Read the model definition and answer for the solid it produces. Units are mm, in the model's axes. Face numbers are marked on the shaded views. A direction names the side the tool comes from. Coordinates: 2 decimals unless noted, no trailing zeros. Answer in a Markdown table with one row per item.
```python
from build123d import *

# Parameters (mm, degrees)
BOSS_EXTRUDE2_DEPTH       = 20
FILLET1_R                 = 30
FILLET2_R                 = 6
SKETCH2_R                 = 7
BOSS_EXTRUDE3_DEPTH       = 65.089952611
SKETCH3_R                 = 4.7625
CUT_EXTRUDE1_DEPTH        = 109.008396677
BOSS_EXTRUDE5_DEPTH       = 26.439795129
BOSS_EXTRUDE5_DEPTH_BACK  = 2
SKETCH6_R                 = 3
SKETCH8_R                 = 5
BOSS_EXTRUDE6_DEPTH       = 77
SKETCH9_R                 = 5
BOSS_EXTRUDE7_DEPTH       = 103.4
BOSS_EXTRUDE8_DEPTH       = 5
BOSS_EXTRUDE9_DEPTH       = 5
CUT_EXTRUDE2_DEPTH        = 2
BOSS_EXTRUDE14_START      = -1
BOSS_EXTRUDE14_DEPTH      = 3
BOSS_EXTRUDE15_DEPTH      = 15
SKETCH23_R                = 10
BOSS_EXTRUDE17_DEPTH      = 20
REVOLVE1_ANGLE            = 15
CIRPATTERN1_COUNT         = 4
CIRPATTERN1_ANGLE         = 273
SKETCH24_R                = 3.175
CUT_EXTRUDE3_DEPTH        = 25.4
SKETCH25_R                = 3.175
CUT_EXTRUDE4_DEPTH        = 25.4
BOSS_EXTRUDE20_DEPTH      = 1.5
BOSS_EXTRUDE20_DEPTH_BACK = 1.5
SKETCH26_W                = 46.97935404
SKETCH26_H                = 6


with BuildPart() as part:
    # Sketch1 → Boss-Extrude2 (new body)
    with BuildSketch(Plane.XY):
        Polygon((0, -8.361996352), (38.1, -8.361996352), (55.47415821, -26.885626298), (38.1, -33.761996352), (0, -33.761996352), (-17.37415821, -26.885626298), align=None)
    extrude(amount=BOSS_EXTRUDE2_DEPTH)

    # Fillet1
    fillet1_edges = [part.edges().sort_by_distance(p)[0] for p in [
        (0, -8.361996352, 10),
        (38.1, -8.361996352, 10),
    ]]
    fillet(fillet1_edges, radius=FILLET1_R)

    # Fillet2
    fillet2_edges = [part.edges().sort_by_distance(p)[0] for p in [
        (46.787079105, -30.323811325, 20),
        (-8.687079105, -30.323811325, 20),
        (46.787079105, -30.323811325, 0),
        (-8.687079105, -30.323811325, 0),
    ]]
    fillet(fillet2_edges, radius=FILLET2_R)

    # Sketch2 → Boss-Extrude3 (add)
    with BuildSketch(Plane.XZ.offset(33.761996352)):
        with Locations(Location((19.05, 10, 0), (0, 0, 180))):
            Circle(SKETCH2_R)
    extrude(amount=BOSS_EXTRUDE3_DEPTH)

    # Sketch3 → Cut-Extrude1 (cut, through all)
    with BuildSketch(Plane.XZ.offset(98.851948963)):
        with Locations((19.05, 10)):
            Circle(SKETCH3_R)
    extrude(amount=-CUT_EXTRUDE1_DEPTH, mode=Mode.SUBTRACT)

    # Sketch6 → Boss-Extrude5 (add, two sides: drawn at the far end of the back side and taken through both)
    with BuildSketch(Plane(origin=(16.71256452, -42.226747224, 0), x_dir=(-0.9298231117187001, -0.36800676748363437, 0), z_dir=(0.36800676748363437, -0.9298231117187001, 0)).offset(-BOSS_EXTRUDE5_DEPTH_BACK)):
        with Locations(Location((-32.344339698, -10, 0), (0, 0, 180))):
            Circle(SKETCH6_R)
    extrude(amount=BOSS_EXTRUDE5_DEPTH + BOSS_EXTRUDE5_DEPTH_BACK)

    # Sketch8 → Boss-Extrude6 (add)
    with BuildSketch(Plane(origin=(26.442588059, -66.811079804, 0), x_dir=(0.9298231117187001, 0.36800676748363437, 0), z_dir=(0.36800676748363437, -0.9298231117187001, 0))):
        with Locations((32.344339698, 10)):
            Circle(SKETCH8_R)
    extrude(amount=BOSS_EXTRUDE6_DEPTH)

    # Sketch9 → Boss-Extrude7 (add)
    with BuildSketch(Plane(origin=(-11.552720348, -29.189643592, 0), x_dir=(-0.9298231117187001, 0.36800676748363437, 0), z_dir=(-0.36800676748363437, -0.9298231117187001, 0))):
        with Locations(Location((-3.081920858, -10, 0), (0, 0, 53.130102354))):
            Circle(SKETCH9_R)
    extrude(amount=BOSS_EXTRUDE7_DEPTH)

    # Sketch11 → Boss-Extrude8 (add)
    with BuildSketch(Plane(origin=(32.698703106, -82.618072703, 0), x_dir=(-0.9298231117187001, -0.36800676748363437, 0), z_dir=(0.36800676748363437, -0.9298231117187001, 0))):
        with BuildLine():
            Line((-32.344339698, -3), (-22.259943936, -3))
            Line((-22.259943936, -3), (-22.259943936, -17))
            Line((-22.259943936, -17), (-32.344339698, -17))
            ThreePointArc((-32.344339698, -17), (-39.344339698, -10), (-32.344339698, -3))
        make_face()
    extrude(amount=BOSS_EXTRUDE8_DEPTH)

    # Sketch15 → Boss-Extrude9 (add)
    with BuildSketch(Plane(origin=(0, -68.851948963, 0), x_dir=(-1, 0, 0), z_dir=(0, -1, 0))):
        with BuildLine():
            Line((-19.05, -3), (-7.185808352, -3))
            Line((-7.185808352, -3), (-7.185808352, -17))
            Line((-7.185808352, -17), (-19.05, -17))
            ThreePointArc((-19.05, -17), (-26.05, -10), (-19.05, -3))
        make_face()
    extrude(amount=BOSS_EXTRUDE9_DEPTH)

    # Sketch17 → Cut-Extrude2 (cut)
    with BuildSketch(Plane(origin=(16.096305264, 15.097459572, 0), x_dir=(0, 0, -1), z_dir=(0.7293749969664987, 0.6841141087568068, 0))):
        with BuildLine():
            Line((-17, -51.560357903), (-17, -29.560357903))
            Line((-17, -29.560357903), (-3, -29.560357903))
            Line((-3, -29.560357903), (-3, -51.560357903))
            ThreePointArc((-3, -51.560357903), (-3.878679656, -53.681678246), (-6, -54.560357903))
            Line((-6, -54.560357903), (-14, -54.560357903))
            ThreePointArc((-14, -54.560357903), (-16.121320344, -53.681678246), (-17, -51.560357903))
        make_face()
    cut_extrude2 = extrude(amount=-CUT_EXTRUDE2_DEPTH, mode=Mode.SUBTRACT)

    # Mirror2: Cut-Extrude2 across plane
    add(cut_extrude2.mirror(Plane(origin=(19.05, -8.361996352, 20), x_dir=(0, 0, 1), z_dir=(-1, 0, 0))), mode=Mode.SUBTRACT)

    # Sketch19 → Boss-Extrude14 (add)
    with BuildSketch(Plane.XY.offset(17).offset(BOSS_EXTRUDE14_START)):
        with BuildLine():
            Line((58.057147373, -72.145843092), (29.272181754, -59.674022052))
            ThreePointArc((29.272181754, -59.674022052), (15.498497411, -59.957615802), (5.959562875, -69.897612467))
            ThreePointArc((5.959562875, -69.897612467), (8.231471856, -75.078194441), (13.412053829, -72.806285459))
            ThreePointArc((13.412053829, -72.806285459), (18.711461905, -67.28406509), (26.363508762, -67.126513006))
            Line((26.363508762, -67.126513006), (55.459651192, -79.705751724))
            ThreePointArc((55.459651192, -79.705751724), (60.391206803, -77.17398758), (58.057147373, -72.145843092))
        make_face()
    boss_extrude14 = extrude(amount=BOSS_EXTRUDE14_DEPTH)

    # Mirror4: Boss-Extrude14 across plane
    add(boss_extrude14.mirror(Plane.XY.offset(10)))

    # Sketch20 → Boss-Extrude15 (add)
    with BuildSketch(Plane.XY.offset(19)):
        Polygon((49.419158693, -77.094244123), (38.542872969, -72.392060841), (40.089263446, -68.815215009), (50.96554917, -73.51739829), align=None)
    extrude(amount=-BOSS_EXTRUDE15_DEPTH)

    # Sketch23 → Boss-Extrude17 (add)
    with BuildSketch(Plane(origin=(34.538736943, -87.267188261, 0), x_dir=(0.9298231117187001, 0.36800676748363437, 0), z_dir=(0.36800676748363437, -0.9298231117187001, 0))):
        with Locations(Location((32.344339698, 10, 0), (0, 0, 143.130102354))):
            Circle(SKETCH23_R)
    extrude(amount=BOSS_EXTRUDE17_DEPTH)

    # Sketch22 → Revolve1 (revolve)
    with BuildSketch(Plane.XY.offset(10)):
        with BuildLine():
            Line((64.613251528, -75.364252363), (73.911482645, -71.684184688))
            add(Edge.make_bspline(
                [(81.271617995, -90.280646922), (84.545728308, -87.915536418), (81.065760473, -79.122886915), (77.585792638, -70.330237413), (73.911482645, -71.684184688)],
                knots=[3.25665709, 3.25665709, 3.25665709, 4.769921199, 4.769921199, 6.283185307, 6.283185307, 6.283185307], degree=2, weights=[1, 0.727152145, 1, 0.727152145, 1]))
            Line((81.271617995, -90.280646922), (71.973386878, -93.960714597))
            Line((71.973386878, -93.960714597), (64.613251528, -75.364252363))
        make_face()
    revolve1 = revolve(axis=Axis((82.112490758, -119.578648703, 10), (-0.3680067674836343, 0.9298231117187002, 0)), revolution_arc=REVOLVE1_ANGLE)

    # CirPattern1: Revolve1 ×4 about axis
    cirpattern1_axis = Axis((82.112490758, -119.578648703, 10), (-0.3680067674836343, 0.9298231117187002, 0))
    for i in range(1, CIRPATTERN1_COUNT):
        add(revolve1.rotate(cirpattern1_axis, i * CIRPATTERN1_ANGLE / (CIRPATTERN1_COUNT - 1)))

    # Sketch24 → Cut-Extrude3 (cut)
    with BuildSketch(Plane(origin=(-49.604620105, -125.333353344, 0), x_dir=(0.9298231117187001, -0.36800676748363437, 0), z_dir=(-0.36800676748363437, -0.9298231117187001, 0))):
        with Locations((3.081920858, 10)):
            Circle(SKETCH24_R)
    extrude(amount=-CUT_EXTRUDE3_DEPTH, mode=Mode.SUBTRACT)

    # Sketch25 → Cut-Extrude4 (cut)
    with BuildSketch(Plane(origin=(54.779109155, -138.407459406, 0), x_dir=(0.9298231117187001, 0.36800676748363437, 0), z_dir=(0.36800676748363437, -0.9298231117187001, 0))):
        with Locations((32.344339698, 10)):
            Circle(SKETCH25_R)
    extrude(amount=-CUT_EXTRUDE4_DEPTH, mode=Mode.SUBTRACT)

    # Sketch26 → Boss-Extrude20 (add, two sides: drawn at the far end of the back side and taken through both)
    with BuildSketch(Plane.XY.offset(10).offset(-BOSS_EXTRUDE20_DEPTH_BACK)):
        with Locations((-10.248504991, -95.851948963)):
            Rectangle(SKETCH26_W, SKETCH26_H)
    extrude(amount=BOSS_EXTRUDE20_DEPTH + BOSS_EXTRUDE20_DEPTH_BACK)


solid = part.part
```
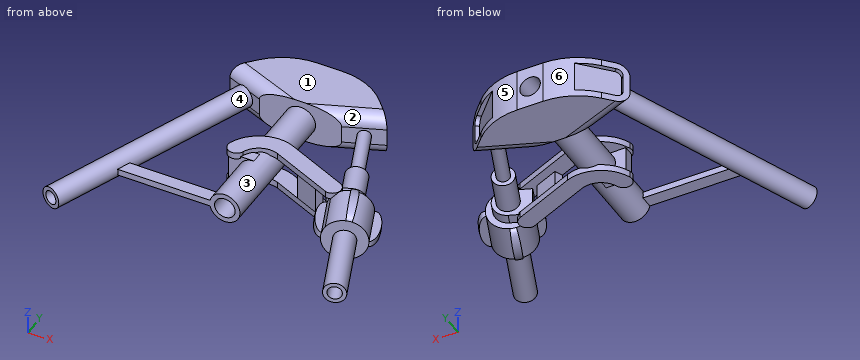
1. Given pin 1 Ø5 at (x, y) = (0.5, -95.5) entering from -Z; pin 2 Ø1.5 at (y, z) = (-108.5, 13) entering from +X; pin 3 Ø23.5 at (x, y) = (31.5, -65.5) entering from -Z, each flat-ended and moving along its own axis, determine where each tip first touches the part or whether it passes through.
A:
| item | result |
|---|---|
| pin 1 | stops at z = 8.5 |
| pin 2 | stops at x = 82.62 |
| pin 3 | stops at z = 1 |
2. The mould has two halves that part along X. Classify the marked faces 4, 5 and 6: pulls with the +X half, pulls with the -X half, needs draft (parallel to the pull), parting line crosses it, or undercut.
A:
| item | result |
|---|---|
| face 4 | undercut |
| face 5 | pulls with the +X half |
| face 6 | pulls with the -X half |
3. Find the intervals of material crossed by probe 1 along Z at (x, y) = (19.05, -78.75); probe 2 along Z at (x, y) = (19.05, -31); probe 3 along Y at (x, z) = (48, 16.5), in increasing order.
A:
| item | result |
|---|---|
| probe 1 | z = 3 to 5.24, 14.76 to 17 |
| probe 2 | z = 0 to 5.24, 14.76 to 20 |
| probe 3 | y = -76.48 to -67.79, -29.26 to -21.84 |
4. A cutting plane is placed at A-A on x = 36. Count the separate pieces of the cut face and the enclosed holes in it, and give its area (3 significant figures).
A:
| item | result |
|---|---|
| separate pieces | 3 |
| enclosed holes | 0 |
| area | 509 mm2 |
5. A tool of negligible diameter and unlimited length cuts with its end or side. For the marked faces 1, 2 and 3, from which of +Z, -Z, +X, -X, +Y, -Y can it reach the whole face along a straight path? Write none if from no direction.
A:
| item | result |
|---|---|
| face 1 | +Z, +X, -X, +Y, -Y |
| face 2 | +Z, +X |
| face 3 | none |
